Work out the finished part from the listing and answer in its coordinate system (mm). Face numbers are marked on the shaded views. A direction names the side the tool comes from. Give positions to 0.01 mm unless a question says otherwise; leave off trailing zeros. Write each loop counter-clockwise with the first axis right and the second up, starting at its lowest first coordinate (ties: lowest second). Pieces come first, ordered by that corner, then holes.
1) Given pin 1 Ø9 at (y, z) = (10, -38) entering from -X; pin 2 Ø12 at (y, z) = (10.5, 16.5) entering from +X; pin 3 Ø3 at (x, y) = (-8.5, 13) entering from +Z; pin 4 Ø3.5 at (y, z) = (12.5, -39.03) entering from -X, each flat-ended and moving along its own axis, determine where each tip first touches the part or whether it passes through.
2) Find section A-A (x = -11.5). Determine the outline of the cut face in (y, z), plus the area to 3 significant figures.
3) Find section D-D (y = 6.25). Determine the outline of the cut face in (x, z), plus the area to 3 significant figures.
4) Determine the mould class of the marked faces 1, 2 and 3 for opening direction Z: pulls with the +Z half, pulls with the -Z half, needs draft (parallel to the pull), parting line crosses it, or undercut.
5) A tool of negligible diameter and unlimited length cuts with its end or side. For the marked faces 4, 5 and 6, from which of +Z, -Z, +X, -X, +Y, -Y can it reach the whole face along a straight path? Write none if from no direction.
6) Find section B-B (y = 12.5). Determine the outline of the cut face in (x, z).
7) Straight lines are drawn through the part: probe 1 along Y at (x, z) = (-5.5, -3); probe 2 along X at (y, z) = (14.25, 0.5); probe 3 along Z at (x, y) = (-11, 11). For each, find the intervals that lie inside material, in ascending order.
8) Find section C-C (z = -25). Determine the outline of the cut face in (x, y).
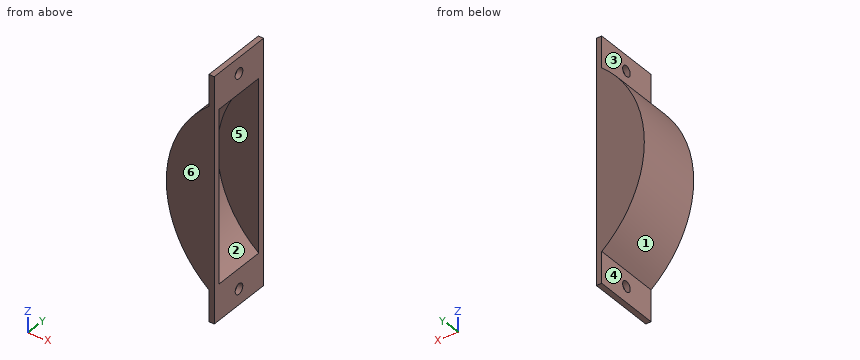
Autodesk Inventor part; units mm, degrees
ref_plane "YZ Plane" through (0, 0, 0) normal (1, 0, 0) x (0, 1, 0)
ref_plane "XZ Plane" through (0, 0, 0) normal (0, 1, 0) x (-1, 0, 0)
ref_plane "XY Plane" through (0, 0, 0) normal (0, 0, 1) x (1, 0, 0)
sketch "Sketch1" plane through (0, 0, 0) normal (0, 1, 0) x (-1, 0, 0)
  circle A0 centre (-25.3492, 0) radius 35.56 construction
  line L0 (0, 84.1375) -> (6.35, 84.1375) construction
  line L1 (6.35, 84.1375) -> (6.35, -68.2625) construction
  line L2 (6.35, -68.2625) -> (0, -68.2625) construction
  line L3 (0, -68.2625) -> (0, 84.1375) construction
  arc A1 (0, -34.8078) -> (0, 34.8078) centre (-25.3492, 0) ccw
  line L4 (0, 34.8078) -> (0, -34.8078)
  point P0 (0, 0)
  point P1 (6.35, 29.1432)
  point P2 (6.35, -29.1432)
  dimension "d0" = 71.12
  dimension "d1" = 25.3492
  dimension "d2" = 6.35
  dimension "d3" = 152.4
  dimension "d4" = 86.12
extrude "Extrusion1" add sketch "Sketch1" along normal blind 25
shell "Shell2" thickness 2.5 removed faces 1 at (0, 8.3333, 11.6026)
sketch "Sketch2" plane through (0, 25, 0) normal (0, 1, 0) x (1, 0, 0)
  line L0 (0, 34.8078) -> (-2, 34.8078)
  line L1 (-2, 34.8078) -> (-2, 44.8078)
  line L2 (-2, 44.8078) -> (0, 44.8078)
  line L3 (0, 44.8078) -> (0, 34.8078)
  line L4 (-2, 34.8078) -> (0, 34.8078)
  line L5 (0.2807, 0) -> (-17.7108, 0) construction
  arc A0 (0, 34.8078) -> (0, -34.8078) centre (25.3492, 0) ccw construction
  line L6 (0, 34.8078) -> (-2, 34.8078)
  line L7 (-2, 34.8078) -> (-2, 33.2594)
  line L8 (-2, 33.2594) -> (0, 33.2594)
  line L9 (0, 33.2594) -> (0, 34.8078)
  line L10 (0, -34.8078) -> (-2, -34.8078)
  line L11 (-2, -34.8078) -> (-2, -44.8078)
  line L12 (-2, -44.8078) -> (0, -44.8078)
  line L13 (0, -44.8078) -> (0, -34.8078)
  line L14 (-2, -34.8078) -> (0, -34.8078)
  arc A1 (0, 34.8078) -> (0, -34.8078) centre (25.3492, 0) ccw construction
  line L15 (0, -34.8078) -> (-2, -34.8078)
  line L16 (-2, -34.8078) -> (-2, -33.2594)
  line L17 (-2, -33.2594) -> (0, -33.2594)
  line L18 (0, -33.2594) -> (0, -34.8078)
  point P0 (0, 0)
  dimension "d9" = 2
  dimension "d10" = 10
  dimension "d15" = 0
  dimension "d16" = 2
extrude "Extrusion2" add sketch "Sketch2" against normal up to surface (25 mm away)
sketch "Sketch3" plane through (-2, 25, 33.2594) normal (-1, 0, 0) x (0, 0, 1)
  circle A0 centre (5.7742, -12.5) radius 1.9304
  line L0 (11.5484, -25) -> (0, -25)
  line L1 (0, 0) -> (11.5484, 0)
  line L2 (0, -25) -> (0, 0)
  line L3 (11.5484, 0) -> (11.5484, -25)
  circle A1 centre (-72.2929, -12.5) radius 1.9304
  line L4 (-78.0671, 0) -> (-78.0671, -25)
  line L5 (-78.0671, 0) -> (-66.5187, 0)
  point P0 (-33.2594, -25)
  dimension "d17" = 3.8608
  dimension "d18" = 25
  dimension "d19" = 12.5
  dimension "d20" = 11.5484
  dimension "d21" = 5.7742
  dimension "d22" = 3.8608
  dimension "d23" = 5.7742
  dimension "d24" = 12.5
extrude "Extrusion3" cut sketch "Sketch3" against normal through all contours A0 | A1
equation "\"d19\" = 0.5 * d18"
equation "\"d21\" = 0.5 * d20"
equation "\"d23\" = d21"
equation "\"d24\" = d19"
properties part number "sprocket cover"
Results:
1. pin 1: stops at x = -2
1. pin 2: stops at x = -8.4
1. pin 3: stops at z = 28.42
1. pin 4: passes through
2. outline: (0, -22.28) - (25, -22.28) - (25, 22.28) - (0, 22.28) - close; hole (2.5, -16.95) - (22.5, -16.95) - (22.5, 16.95) - (2.5, 16.95) - close
2. area: 436 mm2
3. outline: (-2, -44.81) - (0, -44.81) - (0, -31.66) arc R40.56 cw to (0, 31.66) - (0, 44.81) - (-2, 44.81) - (-2, 33.26) arc R43.06 ccw to (-2, -33.26) - close
3. area: 235 mm2
4. face 1: parting line crosses it
4. face 2: undercut
4. face 3: needs draft
5. face 4: -Z, -X, +Y, -Y
5. face 5: +X
5. face 6: +Z, -Z, +X, -X, -Y
6. outline: (-2, -44.81) - (0, -44.81) - (0, -40.96) - (-2, -40.96) - close; (-2, -37.1) - (0, -37.1) - (0, -31.66) arc R40.56 cw to (0, 31.66) - (0, 37.1) - (-2, 37.1) - (-2, 33.26) arc R43.06 ccw to (-2, -33.26) - close; (-2, 40.96) - (0, 40.96) - (0, 44.81) - (-2, 44.81) - close
7. probe 1: y = 0 to 2.5, 22.5 to 25
7. probe 2: x = -17.71 to -15.21
7. probe 3: z = -23.08 to -18, 18 to 23.08
8. outline: (-9.71, 0) - (0, 0) - (0, 2.5) - (-6.59, 2.5) - (-6.59, 22.5) - (0, 22.5) - (0, 25) - (-9.71, 25) - close
